from build123d import *

# Parameters (mm, degrees)
SKETCH1_W                      = 44.45
SKETCH1_H                      = 38.1
BOSS_EXTRUDE1_DEPTH            = 88.9
SKETCH2_W                      = 44.45
SKETCH2_H                      = 6.35
CUT_EXTRUDE1_DEPTH             = 19.05
CUT_EXTRUDE2_REACH             = 95.595
SKETCH3_R                      = 7.9375
CIRPATTERN1_COUNT              = 3
LPATTERN1_COUNT                = 2
LPATTERN1_PITCH                = 9.525
LPATTERN1_COUNT_DIR2           = 2
LPATTERN1_PITCH_DIR2           = 34.925
CBORE_FOR_M3_SHCS1_D           = 3.4
CBORE_FOR_M3_SHCS1_CBORE_D     = 6.5
CBORE_FOR_M3_SHCS1_CBORE_DEPTH = 3
SKETCH11_R                     = 7.9375
CUT_EXTRUDE3_DEPTH             = 12.7
F_8_32_TAPPED_HOLE1_D          = 3.4544
F_8_32_TAPPED_HOLE1_DEPTH      = 19.05
F_8_32_TAPPED_HOLE1_TIP        = 1.037806461
LPATTERN2_COUNT                = 2
LPATTERN2_PITCH                = 25
LPATTERN2_COUNT_DIR2           = 2
LPATTERN2_PITCH_DIR2           = 20


with BuildPart() as part:
    # Sketch1 → Boss-Extrude1 (new body)
    with BuildSketch(Plane(origin=(0, 0, 0), x_dir=(1, 0, 0), z_dir=(0, 1, 0))):
        Rectangle(SKETCH1_W, SKETCH1_H)
    extrude(amount=BOSS_EXTRUDE1_DEPTH)

    # Sketch2 → Cut-Extrude1 (cut)
    with BuildSketch(Plane.XY.offset(19.05)):
        with Locations((0, 3.175)):
            Rectangle(SKETCH2_W, SKETCH2_H)
    extrude(amount=-CUT_EXTRUDE1_DEPTH, mode=Mode.SUBTRACT)

    # Sketch3 → Cut-Extrude2 (cut, up to next)
    with BuildSketch(Plane(origin=(0, 88.9, 0), x_dir=(1, 0, 0), z_dir=(0, 1, 0)), mode=Mode.PRIVATE) as cut_extrude2_sk1:
        with Locations(Location((0, 9.525, 0), (0, 0, 270))):
            Circle(SKETCH3_R)
    cut_extrude2_tool1 = extrude(cut_extrude2_sk1.sketch, amount=-CUT_EXTRUDE2_REACH, mode=Mode.PRIVATE) & part.part
    add(cut_extrude2_tool1.solids().sort_by_distance((0, 88.9, -9.525))[0], mode=Mode.SUBTRACT)

    # Sketch4 → #8-32 Tapped Hole2 (revolve, cut)
    with BuildSketch(Plane(origin=(0, 88.9, 1.5875), x_dir=(0, 0, 1), z_dir=(1, 0, 0))):
        Polygon((0, 0), (0, 13.737806461), (1.7272, 12.7), (1.7272, 0), align=None)
    f_8_32_tapped_hole2 = revolve(axis=Axis((0, 95.25, 1.5875), (0, -1, 0)), mode=Mode.SUBTRACT)

    # CirPattern1: #8-32 Tapped Hole2 ×3 about axis
    cirpattern1_axis = Axis((0, 0, -9.525), (0, 1, 0))
    for i in range(1, CIRPATTERN1_COUNT):
        add(f_8_32_tapped_hole2.rotate(cirpattern1_axis, i * 360 / CIRPATTERN1_COUNT), mode=Mode.SUBTRACT)

    # Sketch6 → #6-32 Tapped Hole1 (revolve, cut)
    with BuildSketch(Plane(origin=(-17.4625, 6.35, 14.2875), x_dir=(0, 0, -1), z_dir=(1, 0, 0))):
        Polygon((0, 0), (0, 18.59269403), (1.35255, 17.78), (1.35255, 0), align=None)
    f_6_32_tapped_hole1 = revolve(axis=Axis((-17.4625, 0, 14.2875), (0, 1, 0)), mode=Mode.SUBTRACT)

    # LPattern1: 6-32 Tapped Hole1 2 × 2
    with Locations(*[(j * LPATTERN1_PITCH_DIR2, 0, -i * LPATTERN1_PITCH) for i in range(LPATTERN1_COUNT) for j in range(LPATTERN1_COUNT_DIR2) if (i, j) != (0, 0)]):
        add(f_6_32_tapped_hole1, mode=Mode.SUBTRACT)

    # CBORE for M3 SHCS1 (through all)
    with Locations(Plane.XY.offset(19.05)):
        with Locations((-12.5, 77.9)):
            cbore_for_m3_shcs1 = CounterBoreHole(CBORE_FOR_M3_SHCS1_D / 2, CBORE_FOR_M3_SHCS1_CBORE_D / 2, CBORE_FOR_M3_SHCS1_CBORE_DEPTH)

    # Sketch11 → Cut-Extrude3 (cut)
    with BuildSketch(Plane.XY.offset(19.05)):
        with Locations((0, 25.4)):
            Circle(SKETCH11_R)
    extrude(amount=-CUT_EXTRUDE3_DEPTH, mode=Mode.SUBTRACT)

    # #8-32 Tapped Hole1
    with Locations(Plane.XY.offset(19.05)):
        with Locations((-11.90625, 25.4), (11.90625, 25.4)):
            Hole(F_8_32_TAPPED_HOLE1_D / 2, depth=F_8_32_TAPPED_HOLE1_DEPTH)
            with Locations((0, 0, -(F_8_32_TAPPED_HOLE1_DEPTH + F_8_32_TAPPED_HOLE1_TIP / 2))):  # 118° drill point
                Cone(0, F_8_32_TAPPED_HOLE1_D / 2, F_8_32_TAPPED_HOLE1_TIP, mode=Mode.SUBTRACT)

    # LPattern2: CBORE for M3 SHCS1 2 × 2
    with Locations(*[(i * LPATTERN2_PITCH, -j * LPATTERN2_PITCH_DIR2, 0) for i in range(LPATTERN2_COUNT) for j in range(LPATTERN2_COUNT_DIR2) if (i, j) != (0, 0)]):
        add(cbore_for_m3_shcs1, mode=Mode.SUBTRACT)


solid = part.part
Here's how the part is built. I have some questions about the finished solid (model axes, mm). A direction names the side the tool comes from. Round coordinates to 2 decimals unless told otherwise and drop trailing zeros. Order: outer loops, then holes, each group sorted by start corner. A loop starts at its lowest first (then second) coordinate and runs counter-clockwise, first axis right, second up. Notation, with made-up numbers: M -39,75.25 L 11,75.25 A38 cw 11,113.25 Z; hole C 68,82 d3. An arc over 180 degrees is marked long. Return JSON: item names as keys, results as strings. Group by question number.
1. If we mould it in two halves opening along Z, with no side actions, what happens to faces 5 (the face through (-18.804, 15.116, 4.939)), 6 (the face through (12.045, 25.134, -0.858)), 7 (the face through (11.795, 74.727, 17.571))? For each: pulls with the +Z half, pulls with the -Z half, needs draft (parallel to the pull), parting line crosses it, or undercut.
2. On a 3-axis mill with a long thin cutter (end or side, diameter ignored), from which of +Z, -Z, +X, -X, +Y, -Y can I reach the whole of each face in a straight line? I mean faces 1 (the face through (0, 3, 0)), 2 (the face through (9.921, 55.922, 17.571)), 3 (the face through (-18.8, 15.1, 14.5)), 4 (the face through (-9.509, 75.342, -14.804)). Say none if no direction works.
3. I'm going to push flat-ended pins straight in: pin 1 Ø3.5 at (x, z) = (17.46, 14.29) entering from -Y; pin 2 Ø4.5 at (x, y) = (12.5, 77.9) entering from +Z; pin 3 Ø12.5 at (x, z) = (0, -9.525) entering from +Y; pin 4 Ø2 at (x, z) = (0, 1.59) entering from +Y. Where does each tip first touch, or does it pass through?
4. If we section it at A-A on y = 57.9: State how many separate pieces and enclosed holes the cut face has, then the cut area to 3 significant figures.
5. If we section it at B-B on z = -5.5: List the corners of the cut face in (x, y) for me (3 decimals), then the cut area to 3 significant figures.
6. Please list where these lines run through material, in increasing order: probe 1 along Y at (x, z) = (12.5, -10); probe 2 along X at (y, z) = (77, 17) (3 decimals); probe 3 along Y at (x, z) = (-12.5, 4).
Reply:
{
 "1": {"face 5": "undercut", "face 6": "pulls with the +Z half", "face 7": "needs draft"},
 "2": {"face 1": "+Z, +X, -X, -Y", "face 2": "+Z", "face 3": "-Y", "face 4": "+Y"},
 "3": {"pin 1": "y = 6.35", "pin 2": "z = 16.05", "pin 3": "through", "pin 4": "y = 75.76"},
 "4": {"separate pieces": "3", "enclosed holes": "1", "area": "1,220 mm^2"},
 "5": {"outline": "M -22.225,0 L -6.841,0 L -6.841,88.9 L -22.225,88.9 Z; M 6.841,0 L 22.225,0 L 22.225,88.9 L 6.841,88.9 Z; hole C -12.5,57.9 d3.4; hole C -12.5,77.9 d3.4; hole C 12.5,57.9 d3.4; hole C 12.5,77.9 d3.4", "area": "2,700 mm^2"},
 "6": {"probe 1": "0 to 56.2, 59.6 to 76.2, 79.6 to 88.9", "probe 2": "-22.225 to -15.623, -9.377 to 9.377, 15.623 to 22.225", "probe 3": "6.35 to 23.78, 27.02 to 56.2, 59.6 to 76.2, 79.6 to 88.9"}
}
